Autodesk Inventor part; units mm, degrees
ref_plane "Work Plane1" through (18.15, 10, -2.5) normal (0, 0, 1) x (1, 0, 0)
ref_plane "YZ Plane" through (0, 0, 0) normal (1, 0, 0) x (0, 1, 0)
ref_plane "XZ Plane" through (0, 0, 0) normal (0, 1, 0) x (-1, 0, 0)
sketch "Sketch1" plane through (0, 0, 0) normal (0, 1, 0) x (-1, 0, 0)
  line L0 (8.15, 22.5) -> (-8.15, 22.5)
  line L1 (-8.15, 22.5) -> (-8.15, -22.5)
  line L2 (-8.15, -22.5) -> (8.15, -22.5)
  line L3 (8.15, -22.5) -> (8.15, 22.5)
  line L4 (8.15, 22.5) -> (-8.15, -22.5) construction
  line L5 (-8.15, 22.5) -> (8.15, -22.5) construction
  line L6 (8.15, 22.5) -> (18.15, 22.5)
  line L7 (18.15, 22.5) -> (18.15, -22.5)
  line L8 (18.15, -22.5) -> (8.15, -22.5)
  line L9 (8.15, -22.5) -> (8.15, 22.5)
  line L10 (-8.15, 22.5) -> (-18.15, 22.5)
  line L11 (-18.15, 22.5) -> (-18.15, -22.5)
  line L12 (-18.15, -22.5) -> (-8.15, -22.5)
  line L13 (-8.15, -22.5) -> (-8.15, 22.5)
  line L14 (-18.15, 22.5) -> (-18.15, 15.65) construction
  line L15 (-18.15, 15.65) -> (18.15, 15.65)
  point P0 (0, 0)
  point P1 (8.15, -22.5)
  point P2 (8.15, 15.65)
  point P3 (-8.15, 15.65)
  dimension "d0" = 16.3
  dimension "d1" = 45
  dimension "d2" = 10
  dimension "d3" = 10
  dimension "d48" = 6.85
extrude "Extrusion1" add sketch "Sketch1" along normal blind 10 contours L15 L7 L8 L3 | L1 L12 L11 L15
sketch "Sketch2" plane through (18.15, 10, 22.5) normal (1, 0, 0) x (0, 0, -1)
  line L0 (0, -10) -> (0, 0) construction
  line L1 (0, -10) -> (11, -10) construction
  line L2 (6.85, -10) -> (45, -10) construction
  line L3 (11, -10) -> (11, -6) construction
  line L4 (11, -10) -> (31, -10) construction
  line L5 (31, -10) -> (31, -6) construction
  circle A0 centre (11, -6) radius 2.25
  circle A1 centre (31, -6) radius 2.25
  point P0 (22.5, -10)
  dimension "d8" = 11
  dimension "d9" = 4
  dimension "d10" = 20
  dimension "d11" = 4
  dimension "d12" = 4.5
extrude "Extrusion3" cut sketch "Sketch2" against normal blind 60
sketch "Sketch3" plane through (0, 0, 0) normal (0, -1, 0) x (1, 0, 0)
  line L0 (8.15, -22.5) -> (-8.15, -22.5) construction
  line L1 (0, -22.5) -> (0, -14.5) construction
  line L2 (-25.15, 10.65) -> (25.15, 10.65)
  line L3 (25.15, 10.65) -> (25.15, -39.65)
  line L4 (25.15, -39.65) -> (-25.15, -39.65)
  line L5 (-25.15, -39.65) -> (-25.15, 10.65)
  line L6 (-25.15, 10.65) -> (25.15, -39.65) construction
  line L7 (25.15, 10.65) -> (-25.15, -39.65) construction
  line L8 (-30.15, 15.65) -> (30.15, 15.65)
  line L9 (30.15, 15.65) -> (30.15, -44.65)
  line L10 (30.15, -44.65) -> (-30.15, -44.65)
  line L11 (-30.15, -44.65) -> (-30.15, 15.65)
  line L12 (-30.15, 15.65) -> (30.15, -44.65) construction
  line L13 (30.15, 15.65) -> (-30.15, -44.65) construction
  point P0 (0, 0)
  dimension "d16" = 8
  dimension "d17" = 50.3
  dimension "d18" = 50.3
  dimension "d19" = 60.3
  dimension "d20" = 60.3
extrude "Extrusion4" add sketch "Sketch3" along normal blind 5 contours L2 L3 L4 L5 | L8 L9 L10 L11
extrude "Extrusion5" add sketch "Sketch3" along normal blind 35
sketch "Sketch4" plane through (30.15, 0, -44.65) normal (0, 0, -1) x (-1, 0, 0)
  circle A0 centre (44.15, -20) radius 2.25
  line L0 (16.15, -20) -> (44.15, -20) construction
  line L1 (0, -35) -> (48, -35) construction
  line L2 (0, -35) -> (0, -20) construction
  circle A1 centre (16.15, -20) radius 2.25
  line L3 (60.3, 0) -> (60.3, -35)
  line L4 (0, 0) -> (0, -35)
  line L5 (60.3, -35) -> (0, -35)
  line L6 (0, -35) -> (0, -5)
  line L7 (0, -5) -> (60.3, -5)
  line L8 (60.3, -5) -> (60.3, -35)
  line L9 (60.3, -35) -> (0, -5) construction
  line L10 (30.15, -20) -> (30.15, -16.3233) construction
  line L11 (30.15, -20) -> (30.15, -23.594) construction
  point P0 (0, -35)
  point P1 (0, -35)
  dimension "d25" = 15
  dimension "d27" = 28
  dimension "d28" = 4.5
  dimension "d29" = 4.5
  dimension "d36" = 30
extrude "Extrusion6" cut sketch "Sketch4" against normal blind 61 contours A0 | A1
sketch "Sketch5" plane through (18.15, 10, -22.5) normal (0, 0, -1) x (-1, 0, 0)
  line L0 (26.3, 0) -> (36.3, 0)
  line L1 (-12, -10) -> (48.3, -10)
  line L2 (36.3, 0) -> (36.3, -15)
  line L3 (36.3, -15) -> (48.3, -15)
  line L4 (48.3, -10) -> (36.3, 0)
  line L5 (0, -10) -> (0, 0)
  line L6 (0, 0) -> (0, -15)
  line L7 (-12, -10) -> (0, -10)
  line L8 (0, -15) -> (-12, -15)
  line L9 (-12, -10) -> (0, 0)
  point P0 (18.15, -10)
  point P1 (36.3, -10)
extrude "Extrusion7" add sketch "Sketch5" against normal blind 8
ref_plane "Work Plane1" through (18.15, 10, -2.5) normal (0, 0, 1) x (1, 0, 0)
sketch "Sketch6" plane through (18.15, 10, -2.5) normal (0, 0, 1) x (1, 0, 0)
  line L0 (-36.3, -10) -> (-48.3, -10)
  line L1 (-36.3, 0) -> (-36.3, -10)
  line L2 (-36.3, 0) -> (-48.3, -10)
  line L3 (12, -10) -> (0, -10)
  line L4 (12, -10) -> (0, 0)
  line L5 (0, -10) -> (0, 0)
  point P0 (-18.15, -10)
extrude "Extrusion8" add sketch "Sketch6" along normal blind 8
fillet "Fillet4" radius 4 2 edges at (19.15, 0, -22.5) (-19.15, 0, -22.5)
properties part number "Suck-brack" material "PBT Plastic"
Can you work these out from the model? Positions are in its coordinate system, mm. A direction names the side the tool comes from. Round coordinates to 2 decimals unless told otherwise and drop trailing zeros. Loops run counter-clockwise (first coordinate to the right, second up) from the corner with the lowest first, then second, coordinate; pieces in that order, holes last. Notation, with made-up numbers: (-12.75, -26.5) -> (23.25, -26.5) arc R21 cw to (23.25, 2.5) -> close; hole circle Ø11 at (22, 87.25). An arc over 180 degrees is marked (long way). Answer in a Markdown table with one row per item.
Item 1: Will these pins go through, and if not, where does the flat tip stop? P1, Ø3.5, axis at x = 27, z = -7.5, coming from the +Y side; P2, Ø2.5, axis at y = 4, z = 11.5, coming from the -X side; P3, Ø5, axis at y = 3.5, z = -6, coming from the -X side; P4, Ø5, axis at x = 23.5, y = 6.5, coming from the -Z side.
Answer block:
| item | result |
|---|---|
| P1 | y = 0 |
| P2 | through |
| P3 | x = -18.15 |
| P4 | z = -22.5 |
Item 2: On a 3-axis mill with a long thin cutter (end or side, diameter ignored), from which of +Z, -Z, +X, -X, +Y, -Y can I reach the whole of each face in a straight line? I mean faces 1 (the flat face through (-24, 0, -8)), 2 (the flat face through (8.15, 5, -5)), 3 (the flat face through (-25.15, -20, -15)), 4 (the flat face through (0, 0, -21)), 5 (the flat face through (-24, 0, 11)). Say none if no direction works.
Answer block:
| item | result |
|---|---|
| face 1 | -X, +Y |
| face 2 | +Z, -Z, +Y |
| face 3 | -Y |
| face 4 | -Z, +Y |
| face 5 | +Z, -X, +Y |
Item 3: Suppose I cut it at D-D, the plane z = -8.5. List the corners of the cut face in (x, y) for me.
Answer block:
| item | result |
|---|---|
| outline | (-30.15, -35) -> (-25.15, -35) -> (-25.15, -5) -> (25.15, -5) -> (25.15, -35) -> (30.15, -35) -> (30.15, 0) -> (18.15, 0) -> (18.15, 1.75) -> (8.15, 1.75) -> (8.15, 0) -> (-8.15, 0) -> (-8.15, 1.75) -> (-18.15, 1.75) -> (-18.15, 0) -> (-30.15, 0) -> close; (-18.15, 6.25) -> (-8.15, 6.25) -> (-8.15, 10) -> (-18.15, 10) -> close; (8.15, 6.25) -> (18.15, 6.25) -> (18.15, 10) -> (8.15, 10) -> close |
Item 4: We'd pull the mould along Z, two halves only. Please class faces 6 (the flat face through (21, 3, 5.5)), 7 (the cylindrical face through (13.22, 4.099, 13.748)), 8 (the cylindrical face through (12.962, -21.996, 13.115)): released by +Z, released by -Z, zero draft, split by the parting line, or undercut.
Answer block:
| item | result |
|---|---|
| face 6 | released by +Z |
| face 7 | undercut |
| face 8 | zero draft |
Item 5: Suppose I cut it at C-C, the plane y = -20. List the corners of the cut face in (x, z) for me.
Answer block:
| item | result |
|---|---|
| outline | (-30.15, -44.65) -> (-16.25, -44.65) -> (-16.25, -39.65) -> (-25.15, -39.65) -> (-25.15, 10.65) -> (-16.25, 10.65) -> (-16.25, 15.65) -> (-30.15, 15.65) -> close; (-11.75, -44.65) -> (11.75, -44.65) -> (11.75, -39.65) -> (-11.75, -39.65) -> close; (-11.75, 10.65) -> (11.75, 10.65) -> (11.75, 15.65) -> (-11.75, 15.65) -> close; (16.25, -44.65) -> (30.15, -44.65) -> (30.15, 15.65) -> (16.25, 15.65) -> (16.25, 10.65) -> (25.15, 10.65) -> (25.15, -39.65) -> (16.25, -39.65) -> close |
Item 6: Suppose I cut it at B-B, the plane x = -14. List the corners of the cut face in (y, z) for me.
Answer block:
| item | result |
|---|---|
| outline | (-35, -44.65) -> (-22.25, -44.65) -> (-22.25, -39.65) -> (-35, -39.65) -> close; (-35, 10.65) -> (-22.25, 10.65) -> (-22.25, 15.65) -> (-35, 15.65) -> close; (-17.75, -44.65) -> (0, -44.65) -> (0, -26.5) arc R4 cw to (4, -22.5) -> (10, -22.5) -> (10, 15.65) -> (-17.75, 15.65) -> (-17.75, 10.65) -> (-5, 10.65) -> (-5, -39.65) -> (-17.75, -39.65) -> close; hole circle Ø4.5 at (4, -8.5); hole circle Ø4.5 at (4, 11.5) |
Item 7: Suppose I cut it at A-A, the plane z = 11.5. List the corners of the cut face in (x, y) for me, plus the area to 3 significant figures.
Answer block:
| item | result |
|---|---|
| outline | (-30.15, -35) -> (30.15, -35) -> (30.15, 0) -> (18.15, 0) -> (18.15, 1.75) -> (8.15, 1.75) -> (8.15, 0) -> (-8.15, 0) -> (-8.15, 1.75) -> (-18.15, 1.75) -> (-18.15, 0) -> (-30.15, 0) -> close; (-18.15, 6.25) -> (-8.15, 6.25) -> (-8.15, 10) -> (-18.15, 10) -> close; (8.15, 6.25) -> (18.15, 6.25) -> (18.15, 10) -> (8.15, 10) -> close; hole circle Ø4.5 at (-14, -20); hole circle Ø4.5 at (14, -20) |
| area | 2,190 mm² |
Item 8: If I drill on probe 1 along X at (y, z) = (-9, -9); probe 2 along Y at (x, z) = (11.5, 11.5); probe 3 along Y at (x, z) = (14, -43.55), over which ranges is the centre line in solid material (lowest first)?
Answer block:
| item | result |
|---|---|
| probe 1 | -30.15 to -25.15, 25.15 to 30.15 |
| probe 2 | -35 to 1.75, 6.25 to 10 |
| probe 3 | -35 to -22.25, -17.75 to 0 |
